```python
from build123d import *

# Parameters (mm, degrees)
SKETCH_3_R      = 1.6
EXTRUDE_1_DEPTH = 1.8


with BuildPart() as part:
    # Sketch 3 → Extrude 1 (new body)
    with BuildSketch(Plane(origin=(0, 0, 0), x_dir=(1, 0, 0), z_dir=(0, 1, 0))):
        with BuildLine():
            Line((-44.29, 110.33), (-23.2864152, 110.33))
            Line((-23.2864152, 110.33), (-23.2864152, 95.33))
            Line((-23.2864152, 95.33), (-29.29, 95.33))
            Line((-29.29, 95.33), (-29.29, 84.723605))
            Line((-29.29, 84.723605), (-29.79, 84.723605))
            Line((-29.79, 84.723605), (-29.79, 82.916395))
            Line((-29.79, 82.916395), (-29.29, 82.916395))
            Line((-29.29, 82.916395), (-29.29, 66.81327125))
            Line((-29.29, 66.81327125), (-32.110172, 66.81327125))
            Line((-32.110172, 66.81327125), (-32.110172, 60.6000312))
            Line((-32.110172, 60.6000312), (-29.29, 60.6000312))
            Line((-29.29, 60.6000312), (-29.29, 39.6))
            Line((-29.29, 39.6), (-31.98, 39.6))
            Line((-31.98, 39.6), (-31.98, 26.44))
            Line((-31.98, 26.44), (-29.29, 26.44))
            Line((-29.29, 26.44), (-29.29, 1.46))
            Line((-29.29, 1.46), (-22.230943256, 1.46))
            ThreePointArc((-22.230943256, 1.46), (-19.05, 3.5), (-15.869056744, 1.46))
            Line((-15.869056744, 1.46), (47.619040111, 1.46))
            ThreePointArc((47.619040111, 1.46), (50.7999886, 3.5000114), (53.980937089, 1.46))
            Line((53.980937089, 1.46), (78.840703168, 1.46))
            ThreePointArc((78.840703168, 1.46), (82.3341, -2.254892), (85.827496832, 1.46))
            Line((85.827496832, 1.46), (178.872422541, 1.46))
            ThreePointArc((178.872422541, 1.46), (182.3339, -2.2230334), (185.795377459, 1.46))
            Line((185.795377459, 1.46), (217.255954056, 1.46))
            ThreePointArc((217.255954056, 1.46), (220.9799886, 4.0000114), (224.704023144, 1.46))
            Line((224.704023144, 1.46), (284.147, 1.46))
            Line((284.147, 1.46), (284.147, 1.811027532))
            ThreePointArc((284.147, 1.811027532), (283.5199886, 3.8100114), (284.147, 5.808995268))
            Line((284.147, 5.808995268), (284.147, 62.771027532))
            ThreePointArc((284.147, 62.771027532), (283.5199886, 64.7700114), (284.147, 66.768995268))
            Line((284.147, 66.768995268), (284.147, 95.33))
            Line((284.147, 95.33), (267.919635947, 95.33))
            ThreePointArc((267.919635947, 95.33), (265.4299886, 94.2900114), (262.940341253, 95.33))
            Line((262.940341253, 95.33), (99.009635947, 95.33))
            ThreePointArc((99.009635947, 95.33), (96.5199886, 94.2900114), (94.030341253, 95.33))
            Line((94.030341253, 95.33), (14.32, 95.33))
            Line((14.32, 95.33), (14.32, 100.33))
            Line((14.32, 100.33), (0.5819962, 100.33))
            Line((0.5819962, 100.33), (0.5819962, 110.33))
            Line((0.5819962, 110.33), (299.56, 110.33))
            Line((299.56, 110.33), (299.56, -12.54))
            Line((299.56, -12.54), (-44.29, -12.54))
            Line((-44.29, -12.54), (-44.29, 110.33))
        make_face()
        with Locations(Location((-31.75, 93.98, 0), (0, 0, 270))):
            Circle(SKETCH_3_R, mode=Mode.SUBTRACT)
        with Locations(Location((20.32, 97.79, 0), (0, 0, 270))):
            Circle(SKETCH_3_R, mode=Mode.SUBTRACT)
        with Locations(Location((96.5199886, 97.7900114, 0), (0, 0, 270))):
            Circle(SKETCH_3_R, mode=Mode.SUBTRACT)
        with Locations(Location((265.4299886, 97.7900114, 0), (0, 0, 270))):
            Circle(SKETCH_3_R, mode=Mode.SUBTRACT)
        with Locations(Location((287.0199886, 64.7700114, 0), (0, 0, 270))):
            Circle(SKETCH_3_R, mode=Mode.SUBTRACT)
        with Locations(Location((287.0199886, 3.8100114, 0), (0, 0, 270))):
            Circle(SKETCH_3_R, mode=Mode.SUBTRACT)
        with Locations(Location((220.9799886, 1.14e-05, 0), (0, 0, 270))):
            Circle(SKETCH_3_R, mode=Mode.SUBTRACT)
        with Locations(Location((50.7999886, 1.14e-05, 0), (0, 0, 270))):
            Circle(SKETCH_3_R, mode=Mode.SUBTRACT)
        with Locations(Location((-19.05, 0, 0), (0, 0, 270))):
            Circle(SKETCH_3_R, mode=Mode.SUBTRACT)
        with Locations(Location((-31.75, 13.97, 0), (0, 0, 270))):
            Circle(SKETCH_3_R, mode=Mode.SUBTRACT)
    extrude(amount=-EXTRUDE_1_DEPTH)


solid = part.part
```
Geometry check sheet. Reference: the model listing, model coordinates, mm. Coordinates: 2 decimals unless noted, no trailing zeros. Write each loop counter-clockwise with the first axis right and the second up, starting at its lowest first coordinate (ties: lowest second). Pieces come first, ordered by that corner, then holes. Notation, with made-up numbers: (2.5, 58.5) -> (31.5, 58.5) arc R22 ccw to (31.5, 72.5) -> close; hole circle Ø8 at (2, 52.25). An arc over 180 degrees is marked (long way). Use CSV: the item, a comma, the result in double quotes. Start each with the question number.
Item 1: Thickness scan on line 1 (Z direction, x = 200, y = -1.15); line 2 (X direction, y = -1.65, z = -25); line 3 (X direction, y = -1.6, z = -37). Record the ranges inside material, lowest first.
Item 2: Cross-section at B-B, the plane z = -51.5. Record the cut outline in (x, y), plus the area to 3 significant figures.
Item 3: Cross-section at D-D, the plane y = -0.65. State how many separate pieces and enclosed holes the cut face has, plus the area to 3 significant figures.
Item 4: Depth check by flat-ended pin: pin 1 Ø2.5 at (x, z) = (287.02, -3.81) entering from +Y. Enter the tip coordinate at first touch or a pass-through.
Item 5: Cross-section at C-C, the plane x = -6. Record the cut outline in (y, z), plus the area to 3 significant figures.
Item 6: Cross-section at A-A, the plane x = 275.5. Record the cut outline in (y, z), plus the area to 3 significant figures.
Answers:
1,line 1,"-110.33 to -95.33, -1.46 to 12.54"
1,line 2,"-44.29 to -29.29, 284.15 to 299.56"
1,line 3,"-44.29 to -31.98, 284.15 to 299.56"
2,outline,"(-44.29, -1.8) -> (-29.29, -1.8) -> (-29.29, 0) -> (-44.29, 0) -> close; (284.15, -1.8) -> (299.56, -1.8) -> (299.56, 0) -> (284.15, 0) -> close"
2,area,"54.7 mm^2"
3,separate pieces,"1"
3,enclosed holes,"10"
3,area,"12,300 mm^2"
4,pin 1,"through"
5,outline,"(-1.8, -1.46) -> (0, -1.46) -> (0, 12.54) -> (-1.8, 12.54) -> close"
5,area,"25.2 mm^2"
6,outline,"(-1.8, -110.33) -> (0, -110.33) -> (0, -95.33) -> (-1.8, -95.33) -> close; (-1.8, -1.46) -> (0, -1.46) -> (0, 12.54) -> (-1.8, 12.54) -> close"
6,area,"52.2 mm^2"
